```python
from build123d import *

# Parameters (mm, degrees)
CHAMFER1_SIZE = 0.5


with BuildPart() as part:
    # Sketch1 → Revolve1 (revolve)
    with BuildSketch(Plane(origin=(0, 0, 0), x_dir=(1, 0, 0), z_dir=(0, 1, 0)), mode=Mode.PRIVATE) as revolve1_sk:
        Polygon((-145, 0), (-145, 8), (-120, 8), (-120, 10), (-114.7, 10), (-114.7, 9.5), (-113.4, 9.5), (-113.4, 10), (-46.5, 10), (-46.5, 12), (46.5, 12), (46.5, 10), (113.4, 10), (113.4, 9.5), (114.7, 9.5), (114.7, 10), (120, 10), (120, 8), (145, 8), (145, 0), align=None)
    revolve(revolve1_sk.sketch.rotate(Axis((-145, 0, 0), (1, 0, 0)), 180), axis=Axis((-145, 0, 0), (1, 0, 0)))

    # Chamfer1
    chamfer1_edges = [part.edges().sort_by_distance(p)[0] for p in [
        (-145, 0, -8),
        (-120, 0, -10),
        (-46.5, 0, -12),
        (46.5, 0, -12),
        (120, 0, -10),
        (145, 0, -8),
    ]]
    chamfer(chamfer1_edges, length=CHAMFER1_SIZE)


solid = part.part
```
CAD build for the part. Positions are in the model's coordinates, mm. A direction names the side the tool comes from. Coordinates: 2 decimals unless noted, no trailing zeros. Write each loop counter-clockwise with the first axis right and the second up, starting at its lowest first coordinate (ties: lowest second). Pieces come first, ordered by that corner, then holes.
(1) Drill centre lines: probe 1 along X at (y, z) = (8.75, 0.5); probe 2 along Y at (x, z) = (62, 0); probe 3 along Z at (x, y) = (83.5, 0.5). Where is each one in solid material? Low to high.
(2) Cut at A-A, the plane x = 50.5. List the corners of the cut face in (y, z), and give its area (3 significant figures).
(3) Flat gauge pins, fed straight in: pin 1 (8 mm diameter, centred on x = 83.5, z = 1.5, fed in from -Y); pin 2 (2 mm diameter, centred on y = 4.5, z = -8, fed in from -X); pin 3 (10 mm diameter, centred on x = 70, y = 5, fed in from +Z). Where does each tip first touch, or does it go through?
(4) Two-plate mould, pull along X, no slides. Class faces 5 (the face through (-132.08, 7.81, -1.73)), 6 (the face through (113.4, 4, 9)), 7 (the face through (145, 0, 0)): +X half, -X half, draft (parallel to the pull), parting line (faces both ways), or undercut.
(5) 3-axis set-ups, long thin cutter, end or side, ignore diameter. For faces 1 (the face through (-120, 7, 4.3)), 2 (the face through (0.644, -3.604, 11.446)), 3 (the face through (114.059, 9.274, -2.059)), 4 (the face through (132.42, 7.81, -1.73)): which of +Z, -Z, +X, -X, +Y, -Y reach the whole face in a straight line?
(6) Cut at B-B, the plane x = -20. List the corners of the cut face in (y, z), and give its area (3 significant figures).
Geometry says:
1. probe 1: x = -120 to 120
1. probe 2: y = -10 to 10
1. probe 3: z = -9.99 to 9.99
2. outline: circle Ø20 at (0, 0)
2. area: 314 mm2
3. pin 1: stops at y = -10
3. pin 2: stops at x = -120
3. pin 3: stops at z = 10
4. face 5: draft
4. face 6: undercut
4. face 7: +X half
5. face 1: -X
5. face 2: +X, -X
5. face 3: none
5. face 4: +X
6. outline: circle Ø24 at (0, 0)
6. area: 452 mm2
